Source: three-view drawing plus pictorial views. Frame: mm from the lowest corner of the part. Coordinates: 2 decimals unless noted, no trailing zeros. Order: outer loops, then holes, each group sorted by start corner. A loop starts at its lowest first (then second) coordinate and runs counter-clockwise, first axis right, second up. Notation, with made-up numbers: (16, 68.5) - (51, 68.5) arc R28 ccw to (51, 103.5) - close; hole circle Ø5 at (29.5, 68.25). An arc over 180 degrees is marked (long way). One line per question, with ' | ' between items.
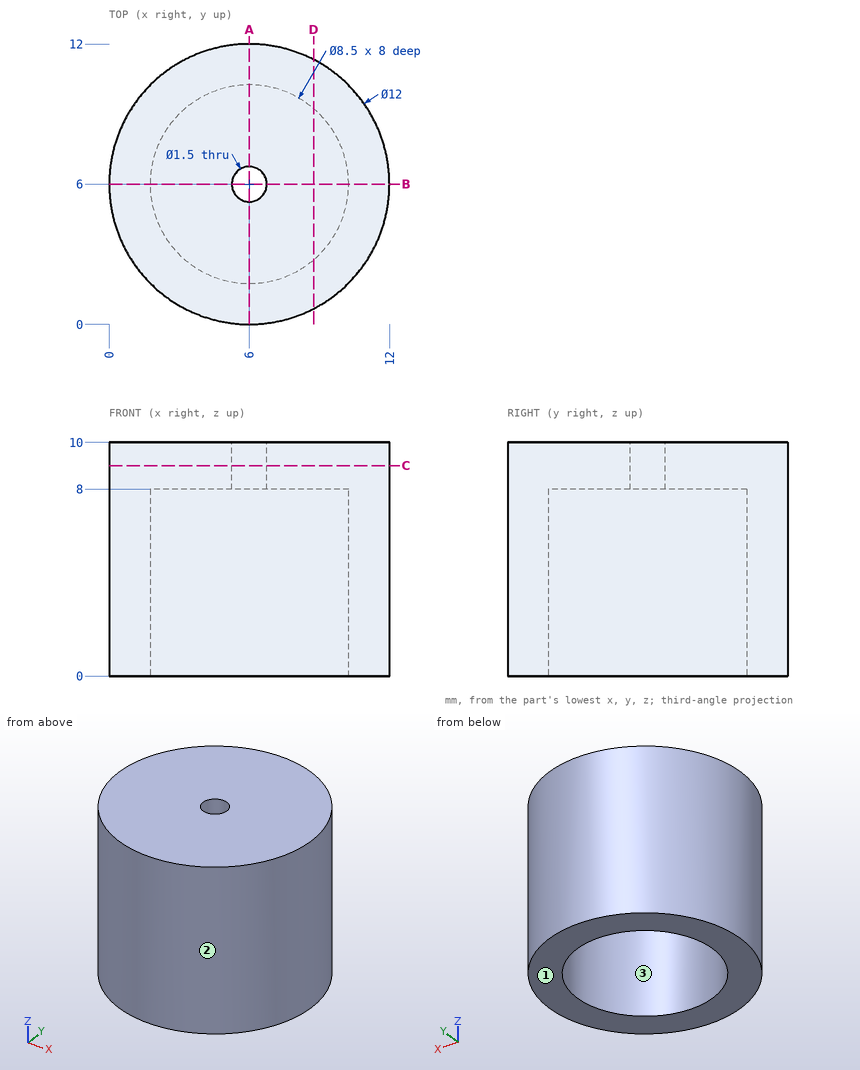
(1) Pull-direction query (Y, two-part tool) for the marked faces 1, 2 and 3; classes: pulls with the +Y half, pulls with the -Y half, needs draft (parallel to the pull), parting line crosses it, or undercut.
Taken from the geometry:
face 1: needs draft | face 2: parting line crosses it | face 3: undercut
(2) Cut plane D-D (x = 8.75). Return the cut outline in (y, z).
Taken from the geometry:
outline: (0.67, 0) - (2.76, 0) - (2.76, 8) - (9.24, 8) - (9.24, 0) - (11.33, 0) - (11.33, 10) - (0.67, 10) - close
(3) Cut plane A-A (x = 6). Return the cut outline in (y, z), and give its area (3 significant figures).
Taken from the geometry:
outline: (0, 0) - (1.75, 0) - (1.75, 8) - (5.25, 8) - (5.25, 10) - (0, 10) - close; (6.75, 8) - (10.25, 8) - (10.25, 0) - (12, 0) - (12, 10) - (6.75, 10) - close | area: 49.0 mm²
(4) Cut plane C-C (z = 9). Return the cut outline in (x, y).
Taken from the geometry:
outline: circle Ø12 at (6, 6); hole circle Ø1.5 at (6, 6)
(5) Material intervals for L1, parallel to Y at x = 6, z = 9.5; L2, parallel to Y at x = 6, z = 4.5; L3, parallel to Z at x = 2.75, y = 6.5, sorted ascending. Write a range as from..to.
Taken from the geometry:
L1: y = 0..5.25, 6.75..12 | L2: y = 0..1.75, 10.25..12 | L3: z = 8..10
(6) Pin query (flat end, axial travel): P1, Ø5, axis at x = 10, z = 7, coming from the -Y side; P2, Ø3, axis at y = 2.5, z = 3.5, coming from the -X side; P3, Ø1, axis at x = 5, z = 4.5, coming from the +Y side. Return the tip coordinate at first contact, or that it passes through.
Taken from the geometry:
P1: stops at y = 0.19 | P2: stops at x = 0.34 | P3: stops at y = 11.98
